The drawing under review shows one solid part. Ordinate dimensions are in mm from its lowest x, y, z. Round coordinates to 2 decimals unless told otherwise and drop trailing zeros. Write each loop counter-clockwise with the first axis right and the second up, starting at its lowest first coordinate (ties: lowest second). Pieces come first, ordered by that corner, then holes.
Item 1: Add section B-B (y = 260.5). Give the boundary of the cut face in (x, z).
Item 2: Add section A-A (x = 100.5). Give the boundary of the cut face in (y, z).
Item 3: Clearance check with flat-ended pins moving along their axes: pin 1 Ø1.5 at (y, z) = (63.5, 1.5) entering from -X; pin 2 Ø1.5 at (y, z) = (327, 2) entering from +X; pin 3 Ø0.9 at (x, z) = (132.5, 1) entering from +Y (1 decimal). State where each tip first meets the part, or that it passes through.
Item 4: To check wall thickness, follow L1, parallel to X at y = 158, z = 2.7; L2, parallel to Y at x = 109, z = 2.45; L3, parallel to Y at x = 82.5, z = 1.15. State the ranges of each line that lie inside material, in increasing order.
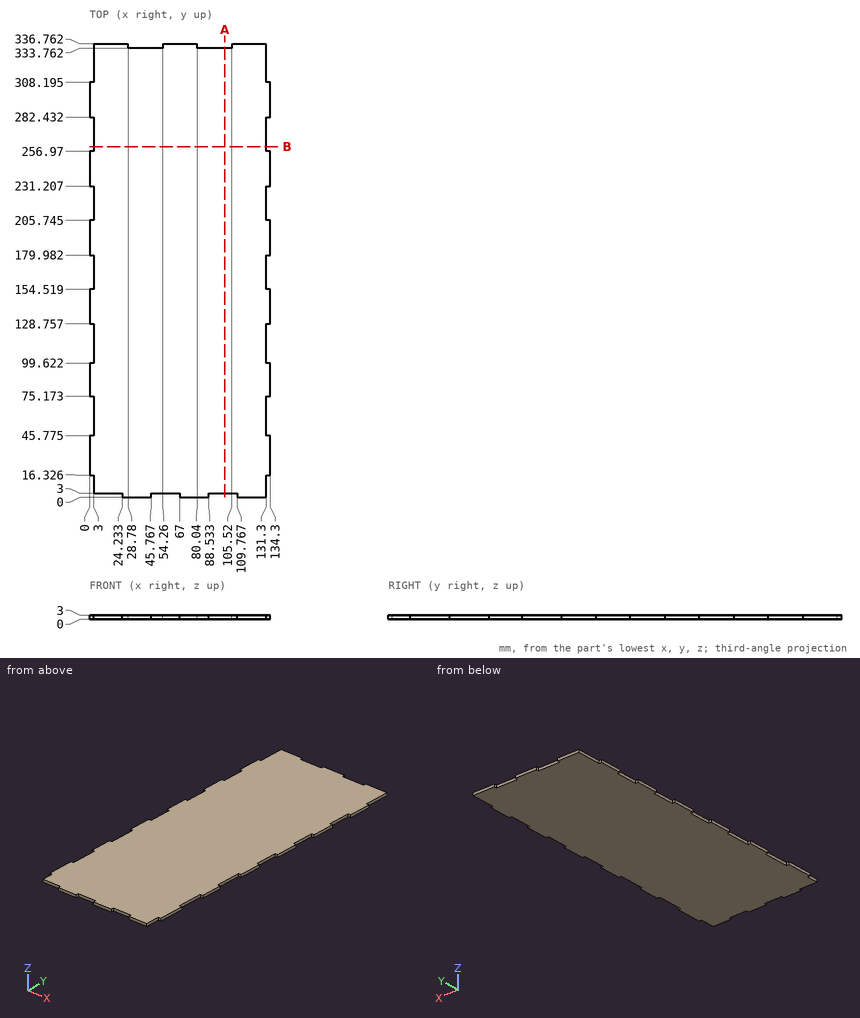
Numbers:
1. outline: (3, 0) - (131.3, 0) - (131.3, 3) - (3, 3) - close
2. outline: (3, 0) - (333.76, 0) - (333.76, 3) - (3, 3) - close
3. pin 1: stops at x = 3
3. pin 2: stops at x = 131.3
3. pin 3: stops at y = 308.2
4. L1: x = 3 to 131.3
4. L2: y = 3 to 336.76
4. L3: y = 0 to 333.76
